```python
from build123d import *

# Parameters (mm, degrees)
SKETCH1_W           = 200
SKETCH1_H           = 500
BOSS_EXTRUDE1_DEPTH = 200
SKETCH2_W           = 70
SKETCH2_H           = 40
BOSS_EXTRUDE2_DEPTH = 75
FILLET1_R           = 25
SKETCH3_R           = 10
CUT_EXTRUDE1_DEPTH  = 75
SKETCH4_W           = 100
SKETCH4_H           = 200
BOSS_EXTRUDE3_DEPTH = 150
SKETCH6_W           = 45
SKETCH6_H           = 25
CUT_EXTRUDE2_DEPTH  = 45
FILLET2_R           = 15


with BuildPart() as part:
    # Sketch1 → Boss-Extrude1 (new body)
    with BuildSketch(Plane(origin=(0, 0, 0), x_dir=(1, 0, 0), z_dir=(0, 1, 0))):
        with Locations((-100, 250)):
            Rectangle(SKETCH1_W, SKETCH1_H)
    extrude(amount=BOSS_EXTRUDE1_DEPTH)

    # Sketch2 → Boss-Extrude2 (add)
    with BuildSketch(Plane(origin=(0, 0, 0), x_dir=(0, 0, -1), z_dir=(1, 0, 0))):
        with Locations((150, 100)):
            Rectangle(SKETCH2_W, SKETCH2_H)
    extrude(amount=BOSS_EXTRUDE2_DEPTH)

    # Fillet1
    fillet1_edges = [part.edges().sort_by_distance(p)[0] for p in [
        (75, 100, -185),
        (75, 100, -115),
    ]]
    fillet(fillet1_edges, radius=FILLET1_R)

    # Sketch3 → Cut-Extrude1 (cut)
    with BuildSketch(Plane(origin=(0, 120, 0), x_dir=(1, 0, 0), z_dir=(0, 1, 0))):
        with Locations(Location((50, 160, 0), (0, 0, 270))):
            Circle(SKETCH3_R)
    extrude(amount=-CUT_EXTRUDE1_DEPTH, mode=Mode.SUBTRACT)

    # Sketch4 → Boss-Extrude3 (add)
    with BuildSketch(Plane(origin=(0, 0, -500), x_dir=(-1, 0, 0), z_dir=(0, 0, -1))):
        with Locations((50, 100)):
            Rectangle(SKETCH4_W, SKETCH4_H)
    extrude(amount=BOSS_EXTRUDE3_DEPTH)

    # Sketch6 → Cut-Extrude2 (cut)
    with BuildSketch(Plane(origin=(75, 0, 0), x_dir=(0, 0, -1), z_dir=(1, 0, 0))):
        with Locations((162.5, 100)):
            Rectangle(SKETCH6_W, SKETCH6_H)
    extrude(amount=-CUT_EXTRUDE2_DEPTH, mode=Mode.SUBTRACT)

    # Fillet2
    fillet2_edges = [part.edges().sort_by_distance(p)[0] for p in [
        (30, 100, -140),
    ]]
    fillet(fillet2_edges, radius=FILLET2_R)


solid = part.part
```
Geometry check sheet. Reference: the model listing, model coordinates, mm. A direction names the side the tool comes from. Give positions to 0.01 mm unless a question says otherwise; leave off trailing zeros. Loops run counter-clockwise (first coordinate to the right, second up) from the corner with the lowest first, then second, coordinate; pieces in that order, holes last. Notation, with made-up numbers: M 23.25,31.25 L 74.25,31.25 A17 cw 74.25,39.25 Z; hole C 77,68 d5. An arc over 180 degrees is marked long. Write item = value, one per line. Start each with the question number.
1. Tool access check on faces 5 (the face through (-151, 99, -500)), 6 (the face through (37, 120, -150)), 7 (the face through (25, 100, -115)), 8 (the face through (19, 100, -185)). Record the directions out of +Z, -Z, +X, -X, +Y, -Y that give a thin tool (end or side, any length) a straight path to the whole face; none if there is none.
2. Section check B-B, the plane z = -566. Enter the section's corners in (x, y).
3. Section check A-A, the plane y = 95.5. Enter the section's corners in (x, z).
4. Section check C-C, the plane y = 48. Enter the section's corners in (x, z), plus the area to 3 significant figures.
5. Draft check along Y on faces 1 (the face through (58, 112.5, -167)), 2 (the face through (37, 80, -150)), 3 (the face through (34.28, 100.18, -144.51)), 4 (the face through (46.17, 116.302, -150.763)). Enter one of: +Y half, -Y half, draft (parallel to the pull), parting line (faces both ways), or undercut.
6. Go/stop test with flat-tipped pins: P1, Ø12.5, axis at x = 57, y = 100, coming from the -Z side; P2, Ø22.5, axis at x = 63.5, z = -165.5, coming from the +Y side; P3, Ø12, axis at x = 35, y = 91, coming from the -Z side. Record where each tip stops, or that it passes through.
7. Section check D-D, the plane z = -428. Enter the section's corners in (x, y), plus the area to 3 significant figures.
8. Thickness scan on probe 1 along X at (y, z) = (116.5, -160); probe 2 along Y at (x, z) = (35.5, -172); probe 3 along Y at (x, z) = (7.5, -155.5). Record the ranges inside material, lowest first.
Values follow:
q1.face_5 = -Z, -X, +Y, -Y
q1.face_6 = +Z, -Z, +X, +Y
q1.face_7 = +Z, +X, +Y, -Y
q1.face_8 = -Z, +X, +Y, -Y
q2.outline = M -100,0 L 0,0 L 0,200 L -100,200 Z
q3.outline = M -200,-500 L -100,-500 L -100,-650 L 0,-650 L 0,-185 L 30,-185 L 30,-155 A15 cw 45,-140 L 75,-140 A25 ccw 50,-115 L 0,-115 L 0,0 L -200,0 Z
q4.outline = M -200,-500 L -100,-500 L -100,-650 L 0,-650 L 0,0 L -200,0 Z
q4.area = 115,000 mm^2
q5.face_1 = undercut
q5.face_2 = -Y half
q5.face_3 = undercut
q5.face_4 = draft
q6.P1 = -140
q6.P2 = 120
q6.P3 = -185
q7.outline = M -200,0 L 0,0 L 0,200 L -200,200 Z
q7.area = 40,000 mm^2
q8.probe_1 = -200 to 40, 60 to 75
q8.probe_2 = 80 to 87.5, 112.5 to 120
q8.probe_3 = 80 to 120
